from build123d import *

# Parameters (mm, degrees)
F0_W     = 110
F0_H     = 90
F1_DEPTH = 3
F2_R     = 5
F4_D     = 5
F5_D     = 5
F6_W     = 14
F6_H     = 18
F6_W_2   = 27
F6_H_2   = 27
F7_DEPTH = 3.001
F8_R     = 2


with BuildPart() as f1:
    # F0 (on Top) → F1 (new body)
    with BuildSketch(Plane.XY):
        Rectangle(F0_W, F0_H)
    extrude(amount=F1_DEPTH)

    # F2
    f2_edges = [f1.edges().sort_by_distance(p)[0] for p in [
        (55, 45, 1.5),
        (55, -45, 1.5),
        (-55, 45, 1.5),
        (-55, -45, 1.5),
    ]]
    fillet(f2_edges, radius=F2_R)

    # F4 (through all)
    with Locations(Plane(origin=(0, 0, 0), x_dir=(1, 0, 0), z_dir=(0, 0, -1))):
        with Locations((-44, -36), (44, -36)):
            Hole(F4_D / 2)

    # F5 (through all)
    with Locations(Plane(origin=(0, 0, 0), x_dir=(1, 0, 0), z_dir=(0, 0, -1))):
        with Locations((-44, 30), (44, 30)):
            Hole(F5_D / 2)

    # F6 (on face) → F7 (cut, through all)
    with BuildSketch(Plane.XY.offset(3)):
        with Locations((-36, 16)):
            Rectangle(F6_W, F6_H)
        with Locations((30.5, 14.5)):
            Rectangle(F6_W_2, F6_H_2)
    extrude(amount=-F7_DEPTH, mode=Mode.SUBTRACT)

    # F8
    f8_edges = [f1.edges().sort_by_distance(p)[0] for p in [
        (-43, 7, 1.5),
        (17, 1, 1.5),
        (-29, 7, 1.5),
        (-43, 25, 1.5),
        (17, 28, 1.5),
        (44, 28, 1.5),
        (44, 1, 1.5),
        (-29, 25, 1.5),
    ]]
    fillet(f8_edges, radius=F8_R)


solid = f1.part
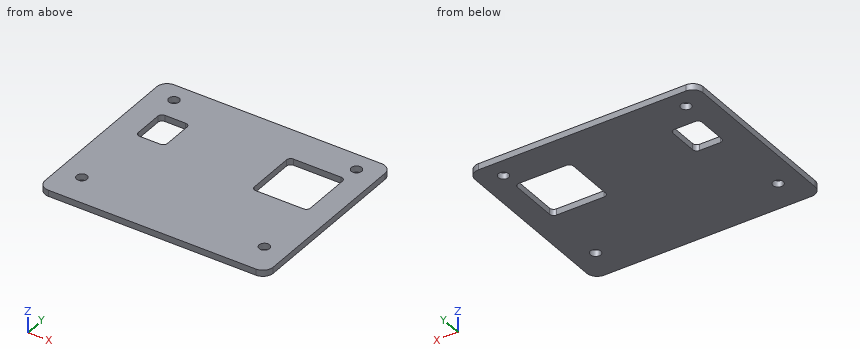
Read the model definition and answer for the solid it produces. Units are mm, in the model's axes. Coordinates: 2 decimals unless noted, no trailing zeros. Loops run counter-clockwise (first coordinate to the right, second up) from the corner with the lowest first, then second, coordinate; pieces in that order, holes last.
Q1. Each of these flat-tipped pins is pushed along its axis until it touches: pin 1 Ø8 at (x, y) = (44, 36) entering from -Z; pin 2 Ø3 at (x, y) = (-44, 36) entering from +Z. Where does it stop, or does it pass through?
Q2. The part is cut by section A-A on x = 28. Write down the section's boundary in (y, z).
Q3. The part is cut by section B-B on y = 13. Write down the section's boundary in (x, z), and give its area (3 significant figures).
Q4. The part is cut by section D-D on y = 36. Write down the section's boundary in (x, z).
Q5. Consider probe 1 along Y at (x, z) = (-44, 1.15); probe 2 along X at (y, z) = (-30, 2.1); probe 3 along Y at (x, z) = (42, 0.8). Determine where each line is inside the solid, lowest interval first.
Q6. The part is cut by section C-C on z = 1.35. Write down the section's boundary in (x, y).
Results below:
1. pin 1: stops at z = 0
1. pin 2: passes through
2. outline: (-45, 0) - (1, 0) - (1, 3) - (-45, 3) - close; (28, 0) - (45, 0) - (45, 3) - (28, 3) - close
3. outline: (-55, 0) - (-43, 0) - (-43, 3) - (-55, 3) - close; (-29, 0) - (17, 0) - (17, 3) - (-29, 3) - close; (44, 0) - (55, 0) - (55, 3) - (44, 3) - close
3. area: 207 mm2
4. outline: (-55, 0) - (-46.5, 0) - (-46.5, 3) - (-55, 3) - close; (-41.5, 0) - (41.5, 0) - (41.5, 3) - (-41.5, 3) - close; (46.5, 0) - (55, 0) - (55, 3) - (46.5, 3) - close
5. probe 1: y = -45 to -32.5, -27.5 to 33.5, 38.5 to 45
5. probe 2: x = -55 to -46.5, -41.5 to 41.5, 46.5 to 55
5. probe 3: y = -45 to -31.5, -28.5 to 1, 28 to 34.5, 37.5 to 45
6. outline: (-55, -40) arc R5 ccw to (-50, -45) - (50, -45) arc R5 ccw to (55, -40) - (55, 40) arc R5 ccw to (50, 45) - (-50, 45) arc R5 ccw to (-55, 40) - close; hole circle Ø5 at (-44, -30); hole circle Ø5 at (-44, 36); hole (-43, 9) arc R2 ccw to (-41, 7) - (-31, 7) arc R2 ccw to (-29, 9) - (-29, 23) arc R2 ccw to (-31, 25) - (-41, 25) arc R2 ccw to (-43, 23) - close; hole (17, 3) arc R2 ccw to (19, 1) - (42, 1) arc R2 ccw to (44, 3) - (44, 26) arc R2 ccw to (42, 28) - (19, 28) arc R2 ccw to (17, 26) - close; hole circle Ø5 at (44, -30); hole circle Ø5 at (44, 36)
